Could you check a few things on this model? Use its own coordinates, in mm. A direction names the side the tool comes from. Give positions to 0.01 mm unless a question says otherwise; leave off trailing zeros. Loops run counter-clockwise (first coordinate to the right, second up) from the corner with the lowest first, then second, coordinate; pieces in that order, holes last. Notation, with made-up numbers: (39.25, -31) -> (69.25, -31) arc R25 ccw to (69.25, -16) -> close; hole circle Ø11 at (58.5, 35.25). An arc over 180 degrees is marked (long way). Write item = value, one per line. Start each with the question number.
1) On a 3-axis mill with a long thin cutter (end or side, diameter ignored), from which of +Z, -Z, +X, -X, +Y, -Y can I reach the whole of each face in a straight line? I mean faces 5 (the face through (9.86, 79.43, 0.6)), 6 (the face through (48.51, 19.4, 3.43)), 7 (the face through (33.913, 36.598, 0.57)). Say none if no direction works.
2) I want a section at A-A (y = 10). List the corners of the cut face in (x, z) for me.
3) I need wall thicknesses on probe 1 along Y at (x, z) = (10, 2.7); probe 2 along X at (y, z) = (32, 3); probe 3 along Y at (x, z) = (9, 3). Which ranges of each line are inside material? Lowest first, please. Write a range as from..to.
4) I'm going to push flat-ended pins straight in: pin 1 Ø1.5 at (x, z) = (61.5, 3) entering from +Y; pin 2 Ø8 at (x, y) = (10, 40) entering from -Z; pin 3 Ø2 at (x, y) = (31, 28) entering from -Z; pin 4 Ø4 at (x, y) = (10, 10) entering from -Z. Where does each tip first touch, or does it pass through?
5) I want a section at B-B (y = 40). Count the separate pieces of the cut face and the enclosed holes in it, and give its area (3 significant figures).
6) If we mould it in two halves opening along X, with no side actions, what happens to faces 1 (the face through (0, 41, 3)), 2 (the face through (19.4, 47.95, 3.43)), 3 (the face through (33.635, 60.145, 0.57)), 4 (the face through (39, 0, 3))? For each: +X half, -X half, draft (parallel to the pull), parting line (faces both ways), or undercut.
from build123d import *

# Parameters (mm, degrees)
F0_R     = 2.5
F1_DEPTH = 4
F3_DEPTH = 25
F4_R     = 2
F5_R     = 1.99999


# Not quite as in the source:
# - a fillet or chamfer is up to 0.001 mm smaller than in the source, because OpenCascade refuses the exact size


with BuildPart() as f1:
    # F0 (on Top) → F1 (new body)
    with BuildSketch(Plane.XY):
        Polygon((0, 80), (0, 0), (80, 0), (80, 20), (20, 80), align=None)
        with Locations((10, 10)):
            Circle(F0_R, mode=Mode.SUBTRACT)
        with Locations((40, 10)):
            Circle(F0_R, mode=Mode.SUBTRACT)
        with Locations((70, 10)):
            Circle(F0_R, mode=Mode.SUBTRACT)
        with Locations((10, 40)):
            Circle(F0_R, mode=Mode.SUBTRACT)
        with Locations((10, 70)):
            Circle(F0_R, mode=Mode.SUBTRACT)
    extrude(amount=F1_DEPTH)

    # F2 (on face) → F3 (cut)
    with BuildSketch(Plane.XY.offset(4)):
        Polygon((44.6966991411, 48.232233047), (20, 72.9289321881), (20, 23.5355339059), align=None)
        Polygon((23.5355339059, 20), (72.9289321881, 20), (48.232233047, 44.6966991411), align=None)
    extrude(amount=-F3_DEPTH, mode=Mode.SUBTRACT)

    # F4
    f4_edges = [f1.edges().sort_by_distance(p)[0] for p in [
        (80, 10, 0),
        (50, 50, 0),
        (10, 80, 0),
        (0, 40, 0),
        (40, 0, 0),
        (72.928932, 20, 2),
        (48.232233, 44.696699, 2),
        (23.535534, 20, 2),
        (44.696699, 48.232233, 2),
        (20, 23.535534, 2),
        (20, 72.928932, 2),
    ]]
    fillet(f4_edges, radius=F4_R)

    # F5 (radius 2 in the source; OpenCascade refuses exactly that, so slightly less here)
    f5_edges = [f1.edges().sort_by_distance(p)[0] for p in [
        (48.232233, 20, 0),
        (20, 48.232233, 0),
        (50, 50, 4),
        (33.34835, 36.883883, 4),
        (59.580583, 33.34835, 4),
    ]]
    fillet(f5_edges, radius=F5_R)


solid = f1.part
Answer list:
q1.face_5 = -Z, +X, -X, +Y
q1.face_6 = +Z
q1.face_7 = -Z
q2.outline = (0, 2) arc R2 ccw to (2, 0) -> (7.5, 0) -> (7.5, 4) -> (0, 4) -> close; (12.5, 0) -> (37.5, 0) -> (37.5, 4) -> (12.5, 4) -> close; (42.5, 0) -> (67.5, 0) -> (67.5, 4) -> (42.5, 4) -> close; (72.5, 0) -> (78, 0) arc R2 ccw to (80, 2) -> (80, 4) -> (72.5, 4) -> close
q3.probe_1 = 0..7.5, 12.5..37.5, 42.5..67.5, 72.5..80
q3.probe_2 = 0..19.73, 28.84..35.16, 61.31..67.62
q3.probe_3 = 0..7.71, 12.29..37.71, 42.29..67.71, 72.29..80
q4.pin_1 = 39.01
q4.pin_2 = 0
q4.pin_3 = 0.1
q4.pin_4 = through
q5.separate_pieces = 4
q5.enclosed_holes = 0
q5.area = 104 mm^2
q6.face_1 = -X half
q6.face_2 = undercut
q6.face_3 = undercut
q6.face_4 = draft
